The drawing under review shows one solid part. Ordinate dimensions are in mm from its lowest x, y, z. A direction names the side the tool comes from. Round coordinates to 2 decimals unless told otherwise and drop trailing zeros. Order: outer loops, then holes, each group sorted by start corner. A loop starts at its lowest first (then second) coordinate and runs counter-clockwise, first axis right, second up. Notation, with made-up numbers: M 3.25,15 L 14.25,15 A23 ccw 14.25,40 Z; hole C 38.25,66.25 d4. An arc over 180 degrees is marked long. Answer as a JSON object with one key per item and string values. Group by question number.
1) Consider section A-A, the plane x = 18.4. Write out the cut boundary in (y, z).
2) Consider section C-C, the plane y = 36. Write out the cut boundary in (x, z).
3) Consider section D-D, the plane x = 23.5. Write out the cut boundary in (y, z).
4) Insertion check: pin 1 Ø3 at (x, y) = (8, 45) entering from +Z; pin 2 Ø6 at (x, y) = (4, 20.5) entering from +Z; pin 3 Ø6 at (y, z) = (29.5, 20) entering from -X. Each pin has a flat end and moves straight along its axis. Give the tip position at first contact, or say it passes through.
5) Consider section B-B, the plane z = 25.4. Write out the cut boundary in (x, y).
6) To check wall thickness, follow line 1 (Y direction, x = 6, z = 29); line 2 (Y direction, x = 19, z = 21.5); line 3 (Z direction, x = 24, y = 62). State the ranges of each line that lie inside material, in increasing order.
7) For the marked faces 1 and 2, list the 3-axis set-ups (+Z, -Z, +X, -X, +Y, -Y) from which the entire face can be reached by the end or side of a thin tool; tool diameter is ignored.
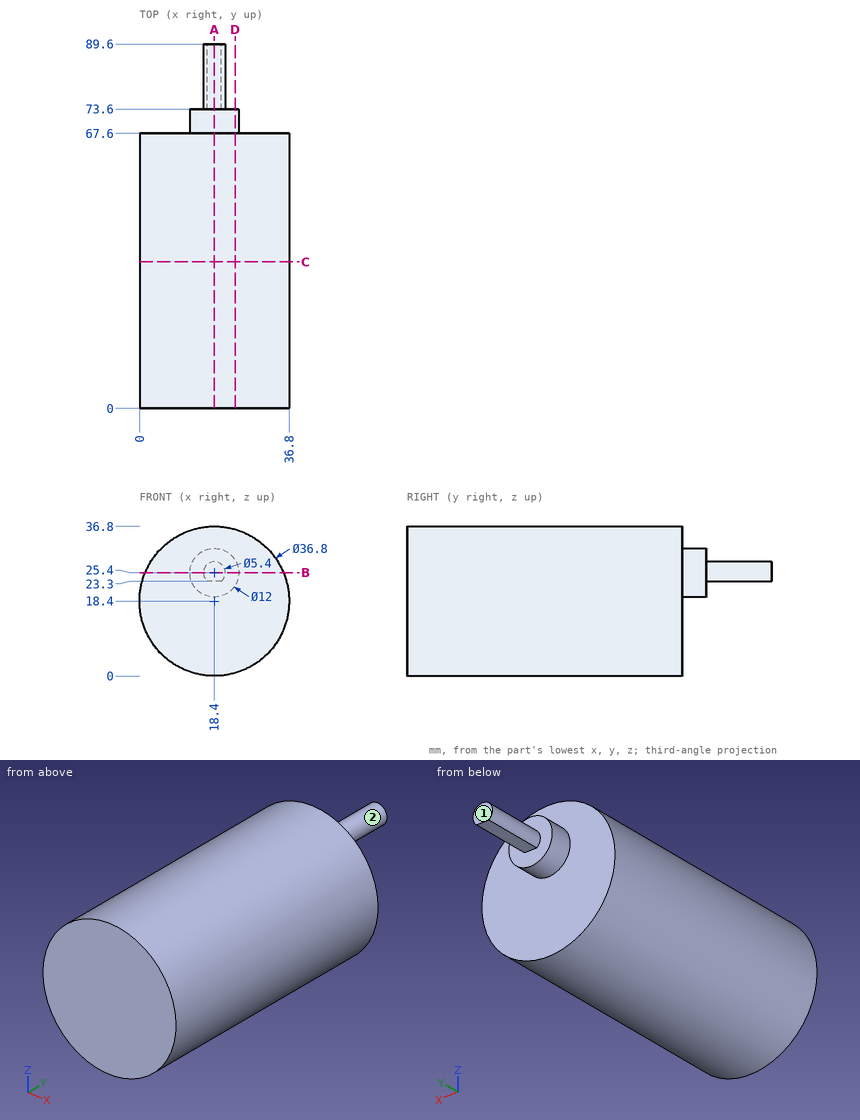
Results list:
{
 "1": {"outline": "M 0,0 L 67.6,0 L 67.6,19.4 L 73.6,19.4 L 73.6,23.3 L 89.6,23.3 L 89.6,28.1 L 73.6,28.1 L 73.6,31.4 L 67.6,31.4 L 67.6,36.8 L 0,36.8 Z"},
 "2": {"outline": "C 18.4,18.4 d36.8"},
 "3": {"outline": "M 0,0.72 L 67.6,0.72 L 67.6,22.24 L 73.6,22.24 L 73.6,28.56 L 67.6,28.56 L 67.6,36.08 L 0,36.08 Z"},
 "4": {"pin 1": "z = 34.5", "pin 2": "z = 32.84", "pin 3": "x = 0"},
 "5": {"outline": "M 1.38,0 L 35.42,0 L 35.42,67.6 L 24.4,67.6 L 24.4,73.6 L 21.1,73.6 L 21.1,89.6 L 15.7,89.6 L 15.7,73.6 L 12.4,73.6 L 12.4,67.6 L 1.38,67.6 Z"},
 "6": {"line 1": "0 to 67.6", "line 2": "0 to 73.6", "line 3": "0.87 to 35.93"},
 "7": {"face 1": "+Z, -Z, +X, -X, +Y", "face 2": "+Y"}
}
